from build123d import *

# Parameters (mm, degrees)
SKETCH1_W           = 120
SKETCH1_H           = 120
BOSS_EXTRUDE1_DEPTH = 25
SKETCH2_R           = 2
CUT_EXTRUDE1_DEPTH  = 172.537167984
SKETCH_1_R          = 57.5
CUT_EXTRUDE_1_DEPTH = 100


with BuildPart() as part:
    # Sketch1 → Boss-Extrude1 (new body)
    with BuildSketch(Plane(origin=(0, 0, 0), x_dir=(1, 0, 0), z_dir=(0, 1, 0))):
        with Locations((60, -60)):
            Rectangle(SKETCH1_W, SKETCH1_H)
    extrude(amount=BOSS_EXTRUDE1_DEPTH)

    # Sketch2 → Cut-Extrude1 (cut, through all)
    with BuildSketch(Plane(origin=(0, 25, 0), x_dir=(1, 0, 0), z_dir=(0, 1, 0))):
        with Locations(Location((7.5, -112.5, 0), (0, 0, 270))):
            Circle(SKETCH2_R)
        with Locations(Location((112.5, -112.5, 0), (0, 0, 270))):
            Circle(SKETCH2_R)
        with Locations(Location((112.5, -7.5, 0), (0, 0, 270))):
            Circle(SKETCH2_R)
        with Locations(Location((7.5, -7.5, 0), (0, 0, 270))):
            Circle(SKETCH2_R)
    extrude(amount=-CUT_EXTRUDE1_DEPTH, mode=Mode.SUBTRACT)

    # 草图1 → 切除-拉伸1 (cut)
    with BuildSketch(Plane(origin=(0, 25, 0), x_dir=(1, 0, 0), z_dir=(0, 1, 0))):
        with Locations(Location((60, -60, 0), (0, 0, 270))):
            Circle(SKETCH_1_R)
    extrude(amount=-CUT_EXTRUDE_1_DEPTH, mode=Mode.SUBTRACT)


solid = part.part
Source: CAD feature listing. Evaluate the final solid. Frame: model axes, mm. Give positions to 0.01 mm unless a question says otherwise; leave off trailing zeros. Loops run counter-clockwise (first coordinate to the right, second up) from the corner with the lowest first, then second, coordinate; pieces in that order, holes last. Notation, with made-up numbers: (67.5, -4) -> (96.5, -4) arc R8 cw to (96.5, 9) -> close; hole circle Ø2 at (-17, 37.5). An arc over 180 degrees is marked (long way). Use a Markdown table: item, result. Add a question column.
1) Section query A-A, the plane y = 6. Return the cut outline in (x, z), then the cut area to 3 significant figures.
2) Line query: line 1 along X through (y, z) = (13, 112.5); line 2 along Z through (x, y) = (59.5, 9.5). Output: solid intervals per line, ascending. Write a range as [from, to].
3) Section query B-B, the plane z = 60. Return the cut outline in (x, y).
4) Section query D-D, the plane z = 7.5. Return the cut outline in (x, y).
5) Pull-direction query (Z, two-part tool) for faces 1 (the face through (25.01, 12.68, 14.37)), 2 (the face through (59, 12, 0)), 3 (the face through (8.852, 12.675, 6.026)), 4 (the face through (120, 12, 61)); classes: +Z half, -Z half, draft (parallel to the pull), parting line (faces both ways), or undercut.
6) Section query C-C, the plane x = 60. Return the cut outline in (y, z).
Numbers:
| question | item | result |
|---|---|---|
| 1 | outline | (0, 0) -> (120, 0) -> (120, 120) -> (0, 120) -> close; hole circle Ø115 at (60, 60); hole circle Ø4 at (7.5, 7.5); hole circle Ø4 at (7.5, 112.5); hole circle Ø4 at (112.5, 7.5); hole circle Ø4 at (112.5, 112.5) |
| 1 | area | 3,960 mm2 |
| 2 | line 1 | x = [0, 5.5], [9.5, 36.55], [83.45, 110.5], [114.5, 120] |
| 2 | line 2 | z = [0, 2.5], [117.5, 120] |
| 3 | outline | (0, 0) -> (2.5, 0) -> (2.5, 25) -> (0, 25) -> close; (117.5, 0) -> (120, 0) -> (120, 25) -> (117.5, 25) -> close |
| 4 | outline | (0, 0) -> (5.5, 0) -> (5.5, 25) -> (0, 25) -> close; (9.5, 0) -> (36.55, 0) -> (36.55, 25) -> (9.5, 25) -> close; (83.45, 0) -> (110.5, 0) -> (110.5, 25) -> (83.45, 25) -> close; (114.5, 0) -> (120, 0) -> (120, 25) -> (114.5, 25) -> close |
| 5 | face 1 | undercut |
| 5 | face 2 | -Z half |
| 5 | face 3 | undercut |
| 5 | face 4 | draft |
| 6 | outline | (0, 0) -> (25, 0) -> (25, 2.5) -> (0, 2.5) -> close; (0, 117.5) -> (25, 117.5) -> (25, 120) -> (0, 120) -> close |
